Source: CAD feature listing. Evaluate the final solid. Frame: model axes, mm. A direction names the side the tool comes from. Give positions to 0.01 mm unless a question says otherwise; leave off trailing zeros. Write each loop counter-clockwise with the first axis right and the second up, starting at its lowest first coordinate (ties: lowest second). Pieces come first, ordered by that corner, then holes. Notation, with made-up numbers: (50, 88.5) -> (71, 88.5) arc R14 ccw to (71, 92.5) -> close; hole circle Ø11 at (7, 9). An arc over 180 degrees is marked (long way). Write item = value, one per line.
from build123d import *

# Parameters (mm, degrees)
SKETCH_1_R          = 3
EXTRUDE_1_DEPTH     = 1
SKETCH_2_R          = 1.5
EXTRUDE_2_DEPTH     = 10
CUT_EXTRUDE_1_DEPTH = 1
FILLET_1_SIZE       = 0.5
FILLET_1_SIZE_2     = 1
CHAMFER_1_SIZE      = 0.5


with BuildPart() as part:
    # 草图1 → 凸台-拉伸1 (new body)
    with BuildSketch(Plane(origin=(0, 0, 0), x_dir=(1, 0, 0), z_dir=(0, 1, 0))):
        with Locations(Location((0, 0, 0), (0, 0, 270))):
            Circle(SKETCH_1_R)
    extrude(amount=EXTRUDE_1_DEPTH)

    # 草图2 → 凸台-拉伸2 (add)
    with BuildSketch(Plane(origin=(0, 1, 0), x_dir=(1, 0, 0), z_dir=(0, 1, 0))):
        with Locations(Location((0, 0, 0), (0, 0, 270))):
            Circle(SKETCH_2_R)
    extrude(amount=EXTRUDE_2_DEPTH)

    # 草图3 → 切除-拉伸1 (cut)
    with BuildSketch(Plane.XZ):
        Polygon((0, 1.154700538), (-1, 0.577350269), (-1, -0.577350269), (0, -1.154700538), (1, -0.577350269), (1, 0.577350269), align=None)
    extrude(amount=-CUT_EXTRUDE_1_DEPTH, mode=Mode.SUBTRACT)

    # 圆角1
    # an asymmetric fillet: 1, 0.5 mm, written as the material it takes off along each edge
    with BuildSketch(Plane(origin=(0, 0, 0), x_dir=(0, 0, 1), z_dir=(-1, 0, 0))) as fillet_1_piece_1:
        with BuildLine():
            Bezier((3, FILLET_1_SIZE), (3, 0), (3 - FILLET_1_SIZE_2, 0), weights=[1, 0.707106781, 1])
            Line((3 - FILLET_1_SIZE_2, 0), (3, 0))
            Line((3, 0), (3, FILLET_1_SIZE))
        make_face()
    revolve(axis=Axis((0, 0, 0), (0, 1, 0)), mode=Mode.SUBTRACT)

    # 倒角1
    chamfer_1_edges = [part.edges().sort_by_distance(p)[0] for p in [
        (0, 11, -1.5),
    ]]
    chamfer(chamfer_1_edges, length=CHAMFER_1_SIZE)


solid = part.part
1) Access query for faces 1 (the flat face through (0, 11, 0)), 2 (the cylindrical face through (0.45, 5.68, 1.43)), 3 (the flat face through (0, 1, 0)). Directions: +Z, -Z, +X, -X, +Y, -Y. A direction counts if a zero-diameter tool reaches every point of the face in a straight line with its end or side. Return the directions, or none.
Computed:
face_1 = +Z, -Z, +X, -X, +Y
face_2 = +Y
face_3 = -Y
2) Contact query for flat-ended pins moving along their axis: pin 1 (3 mm diameter, centred on y = 6, z = 0.5, fed in from -X); pin 2 (1 mm diameter, centred on x = -1, z = -2, fed in from +Y). Output: stop coordinate, or through.
Computed:
pin_1 = -1.5
pin_2 = 1
3) Draft query along Z for faces 4 (the flat face through (-1.3, 1, 1.3)), 5 (the cylindrical face through (0.9, 0.75, 2.86)), 6 (the flat face through (1, 0.5, 0)). Return one class per face: pulls with the +Z half, pulls with the -Z half, needs draft (parallel to the pull), parting line crosses it, or undercut.
Computed:
face_4 = needs draft
face_5 = parting line crosses it
face_6 = undercut
4) Material intervals for L1, parallel to Y at x = -1.75, z = -1; L2, parallel to Y at x = 0, z = 0.75; L3, parallel to X at y = 8.5, z = 0.25, sorted ascending.
Computed:
L1 = 0 to 1
L2 = 1 to 11
L3 = -1.48 to 1.48
5) Cut plane A-A (y = 5.75). Return the cut outline in (x, z), then the cut area to 3 significant figures.
Computed:
outline = circle Ø3 at (0, 0)
area = 7.07 mm²
